Geometry: final body of the model. Coordinates: model frame, mm. A direction names the side the tool comes from. Give positions to 0.01 mm unless a question says otherwise; leave off trailing zeros. Use one line per item in the form item = value.
```python
from build123d import *

# Parameters (mm, degrees)
SKETCH_1_R      = 2.103037388
EXTRUDE_1_DEPTH = 330


with BuildPart() as part:
    # 草图1 → 凸台-拉伸1 (new body)
    with BuildSketch(Plane.XY):
        with BuildLine():
            Line((-32.248557314, -0.229845073), (-32.248557314, -1.030984477))
            Line((-32.248557314, -1.030984477), (-33.250003689, -1.030984477))
            Line((-33.250003689, -1.030984477), (-33.250003689, -6.238394755))
            ThreePointArc((-33.250003689, -6.238394755), (-32.949991565, -6.938952391), (-32.24382973, -7.225524788))
            Line((-32.24382973, -7.225524788), (-27.078556151, -7.225524788))
            Line((-27.078556151, -7.225524788), (-27.078556151, -6.224078413))
            Line((-27.078556151, -6.224078413), (-26.277399051, -6.224078413))
            Line((-26.277399051, -6.224078413), (-26.277399051, -5.212715786))
            Line((-26.277399051, -5.212715786), (-29.27300496, -5.212715786))
            Line((-29.27300496, -5.212715786), (-29.27300496, -4.211495229))
            Line((-29.27300496, -4.211495229), (-26.279632969, -1.225390538))
            Line((-26.279632969, -1.225390538), (-20.24902045, -1.225390538))
            Line((-20.24902045, -1.225390538), (-17.255648459, -4.211495229))
            Line((-17.255648459, -4.211495229), (-17.255648459, -5.212715786))
            Line((-17.255648459, -5.212715786), (-20.251254368, -5.212715786))
            Line((-20.251254368, -5.212715786), (-20.251254368, -6.224078413))
            Line((-20.251254368, -6.224078413), (-19.450097268, -6.224078413))
            Line((-19.450097268, -6.224078413), (-19.450097268, -7.225524788))
            Line((-19.450097268, -7.225524788), (-7.064233131, -7.225524788))
            Line((-7.064233131, -7.225524788), (-7.064233131, -6.224078413))
            Line((-7.064233131, -6.224078413), (-6.263076031, -6.224078413))
            Line((-6.263076031, -6.224078413), (-6.263076031, -5.212715786))
            Line((-6.263076031, -5.212715786), (-9.25868194, -5.212715786))
            Line((-9.25868194, -5.212715786), (-9.25868194, -4.211495229))
            Line((-9.25868194, -4.211495229), (-6.265309949, -1.225390538))
            Line((-6.265309949, -1.225390538), (-0.234697429, -1.225390538))
            Line((-0.234697429, -1.225390538), (2.758674561, -4.211495229))
            Line((2.758674561, -4.211495229), (2.758674561, -5.212715786))
            Line((2.758674561, -5.212715786), (-0.236931348, -5.212715786))
            Line((-0.236931348, -5.212715786), (-0.236931348, -6.224078413))
            Line((-0.236931348, -6.224078413), (0.564225752, -6.224078413))
            Line((0.564225752, -6.224078413), (0.564225752, -7.225524788))
            Line((0.564225752, -7.225524788), (12.945482254, -7.225524788))
            Line((12.945482254, -7.225524788), (12.945482254, -6.219120287))
            Line((12.945482254, -6.219120287), (13.751246989, -6.219120287))
            Line((13.751246989, -6.219120287), (13.751246989, -5.212715786))
            Line((13.751246989, -5.212715786), (10.755641081, -5.212715786))
            Line((10.755641081, -5.212715786), (10.755641081, -4.211495229))
            Line((10.755641081, -4.211495229), (13.749013071, -1.225390538))
            Line((13.749013071, -1.225390538), (19.779625591, -1.225390538))
            Line((19.779625591, -1.225390538), (22.772997581, -4.211495229))
            Line((22.772997581, -4.211495229), (22.772997581, -5.212715786))
            Line((22.772997581, -5.212715786), (19.772784037, -5.212715786))
            Line((19.772784037, -5.212715786), (19.772784037, -6.219120287))
            Line((19.772784037, -6.219120287), (20.573941137, -6.219120287))
            Line((20.573941137, -6.219120287), (20.573941137, -7.225524788))
            Line((20.573941137, -7.225524788), (25.743822351, -7.225524788))
            ThreePointArc((25.743822351, -7.225524788), (26.449984187, -6.938952391), (26.749996311, -6.238394755))
            Line((26.749996311, -6.238394755), (26.749996311, -1.030984477))
            Line((26.749996311, -1.030984477), (25.748549936, -1.030984477))
            Line((25.748549936, -1.030984477), (25.748549936, -0.229827377))
            Line((25.748549936, -0.229827377), (24.761302481, -0.229827377))
            Line((24.761302481, -0.229827377), (24.761302481, -3.234203038))
            Line((24.761302481, -3.234203038), (23.759856106, -3.234203038))
            Line((23.759856106, -3.234203038), (20.770104831, -0.237175589))
            Line((20.770104831, -0.237175589), (20.770104831, 5.786126014))
            Line((20.770104831, 5.786126014), (23.759856106, 8.783153462))
            Line((23.759856106, 8.783153462), (24.761302481, 8.783153462))
            Line((24.761302481, 8.783153462), (24.761302481, 5.778777801))
            Line((24.761302481, 5.778777801), (25.748549936, 5.778777801))
            Line((25.748549936, 5.778777801), (25.748549936, 6.579934901))
            Line((25.748549936, 6.579934901), (26.749996311, 6.579934901))
            Line((26.749996311, 6.579934901), (26.749996311, 11.768212512))
            ThreePointArc((26.749996311, 11.768212512), (26.456722319, 12.481138347), (25.743822351, 12.774475212))
            Line((25.743822351, 12.774475212), (20.573941137, 12.774475212))
            Line((20.573941137, 12.774475212), (20.573941137, 11.768070711))
            Line((20.573941137, 11.768070711), (19.772784037, 11.768070711))
            Line((19.772784037, 11.768070711), (19.772784037, 10.761666211))
            Line((19.772784037, 10.761666211), (22.772997581, 10.761666211))
            Line((22.772997581, 10.761666211), (22.772997581, 9.760445653))
            Line((22.772997581, 9.760445653), (19.779625591, 6.774340962))
            Line((19.779625591, 6.774340962), (13.749013071, 6.774340962))
            Line((13.749013071, 6.774340962), (10.755641081, 9.760445653))
            Line((10.755641081, 9.760445653), (10.755641081, 10.761666211))
            Line((10.755641081, 10.761666211), (13.746639354, 10.761666211))
            Line((13.746639354, 10.761666211), (13.746639354, 11.768070711))
            Line((13.746639354, 11.768070711), (12.945482254, 11.768070711))
            Line((12.945482254, 11.768070711), (12.945482254, 12.774475212))
            Line((12.945482254, 12.774475212), (0.564225752, 12.774475212))
            Line((0.564225752, 12.774475212), (0.564225752, 11.773028837))
            Line((0.564225752, 11.773028837), (-0.236931348, 11.773028837))
            Line((-0.236931348, 11.773028837), (-0.236931348, 10.761666211))
            Line((-0.236931348, 10.761666211), (2.758674561, 10.761666211))
            Line((2.758674561, 10.761666211), (2.758674561, 9.760445653))
            Line((2.758674561, 9.760445653), (-0.234697429, 6.774340962))
            Line((-0.234697429, 6.774340962), (-6.265309949, 6.774340962))
            Line((-6.265309949, 6.774340962), (-9.25868194, 9.760445653))
            Line((-9.25868194, 9.760445653), (-9.25868194, 10.761666211))
            Line((-9.25868194, 10.761666211), (-6.263076031, 10.761666211))
            Line((-6.263076031, 10.761666211), (-6.263076031, 11.773028837))
            Line((-6.263076031, 11.773028837), (-7.064233131, 11.773028837))
            Line((-7.064233131, 11.773028837), (-7.064233131, 12.774475212))
            Line((-7.064233131, 12.774475212), (-19.450097268, 12.774475212))
            Line((-19.450097268, 12.774475212), (-19.450097268, 11.773028837))
            Line((-19.450097268, 11.773028837), (-20.251254368, 11.773028837))
            Line((-20.251254368, 11.773028837), (-20.251254368, 10.761666211))
            Line((-20.251254368, 10.761666211), (-17.255648459, 10.761666211))
            Line((-17.255648459, 10.761666211), (-17.255648459, 9.760445653))
            Line((-17.255648459, 9.760445653), (-20.24902045, 6.774340962))
            Line((-20.24902045, 6.774340962), (-26.279632969, 6.774340962))
            Line((-26.279632969, 6.774340962), (-29.27300496, 9.760445653))
            Line((-29.27300496, 9.760445653), (-29.27300496, 10.761666211))
            Line((-29.27300496, 10.761666211), (-26.277399051, 10.761666211))
            Line((-26.277399051, 10.761666211), (-26.277399051, 11.773028837))
            Line((-26.277399051, 11.773028837), (-27.078556151, 11.773028837))
            Line((-27.078556151, 11.773028837), (-27.078556151, 12.774475212))
            Line((-27.078556151, 12.774475212), (-32.24382973, 12.774475212))
            ThreePointArc((-32.24382973, 12.774475212), (-32.956729698, 12.481138347), (-33.250003689, 11.768212512))
            Line((-33.250003689, 11.768212512), (-33.250003689, 6.560802234))
            Line((-33.250003689, 6.560802234), (-32.248557314, 6.560802234))
            Line((-32.248557314, 6.560802234), (-32.248557314, 5.759645134))
            Line((-32.248557314, 5.759645134), (-31.261309859, 5.759645134))
            Line((-31.261309859, 5.759645134), (-31.261309859, 8.764020795))
            Line((-31.261309859, 8.764020795), (-30.259863484, 8.764020795))
            Line((-30.259863484, 8.764020795), (-27.27011221, 5.766993347))
            Line((-27.27011221, 5.766993347), (-27.27011221, -0.237175589))
            Line((-27.27011221, -0.237175589), (-30.259863484, -3.234203038))
            Line((-30.259863484, -3.234203038), (-31.261309859, -3.234203038))
            Line((-31.261309859, -3.234203038), (-31.261309859, -0.229845073))
            Line((-31.261309859, -0.229845073), (-32.248557314, -0.229845073))
        make_face()
        with Locations((-3.250003689, 2.774475212)):
            Circle(SKETCH_1_R, mode=Mode.SUBTRACT)
        with Locations((-23.250003689, 2.774475212)):
            Circle(SKETCH_1_R, mode=Mode.SUBTRACT)
        with Locations((16.749996311, 2.774475212)):
            Circle(SKETCH_1_R, mode=Mode.SUBTRACT)
        Polygon((-19.258541209, 5.786126014), (-19.258541209, -0.237175589), (-15.26734356, -4.238086639), (-15.26734356, -5.22228212), (-11.246986839, -5.22228212), (-11.246986839, -4.238086639), (-7.25578919, -0.237175589), (-7.25578919, 2.774475212), (-7.25578919, 5.786126014), (-11.246986839, 9.787037063), (-11.246986839, 10.771232544), (-15.26734356, 10.771232544), (-15.26734356, 9.787037063), align=None, mode=Mode.SUBTRACT)
        Polygon((4.74697946, -5.22228212), (8.767336181, -5.22228212), (8.767336181, -4.238086639), (12.758533831, -0.237175589), (12.758533831, 2.774475212), (12.758533831, 5.786126014), (8.767336181, 9.787037063), (8.767336181, 10.771232544), (4.74697946, 10.771232544), (4.74697946, 9.787037063), (0.755781811, 5.786126014), (0.755781811, 2.774475212), (0.755781811, -0.237175589), (4.74697946, -4.238086639), align=None, mode=Mode.SUBTRACT)
    extrude(amount=EXTRUDE_1_DEPTH)


solid = part.part
```
(1) Cut plane A-A (z = 140). Give the number of separate pieces and of enclosed holes in the cut face, plus the area to 3 significant figures.
Solution:
separate_pieces = 1
enclosed_holes = 5
area = 448 mm2
(2) Pin query (flat end, axial travel): P1, Ø0.6, axis at x = -6.5, z = 119.5, coming from the +Y side; P2, Ø6, axis at y = 3, z = 238.5, coming from the +X side; P3, Ø1.5, axis at x = -26, z = 156.5, coming from the -Y side. Return the tip coordinate at first contact, or that it passes through.
Solution:
P1 = 11.77
P2 = 25.75
P3 = -6.22
(3) Pull-direction query (X, two-part tool) for faces 1 (the face through (-23, 6.774, 163)), 2 (the face through (-27.27, 3, 163)), 3 (the face through (-13, -7.226, 163)), 4 (the face through (26.75, -4, 163)); classes: released by +X, released by -X, zero draft, split by the parting line, or undercut.
Solution:
face_1 = undercut
face_2 = released by -X
face_3 = zero draft
face_4 = released by +X
(4) Material intervals for L1, parallel to X at y = 3, z = 134; L2, parallel to X at y = 5.5, z = 79; L3, parallel to Y at x = -13, z = 275, sorted ascending. Write a range as from..to.
Solution:
L1 = -27.27..-25.34, -21.16..-19.26, -7.26..-5.34, -1.16..0.76, 12.76..14.66, 18.84..20.77
L2 = -27.27..-19.26, -7.26..0.76, 12.76..20.77
L3 = -7.23..-5.22, 10.77..12.77
(5) Access query for faces 5 (the face through (-7.256, 3, 163)), 6 (the face through (-3, 6.774, 163)), 7 (the face through (-23, -1.225, 163)), 8 (the face through (20.77, 3, 163)). Directions: +Z, -Z, +X, -X, +Y, -Y. A direction counts if a zero-diameter tool reaches every point of the face in a straight line with its end or side. Return the directions, or none.
Solution:
face_5 = +Z, -Z
face_6 = +Z, -Z, +Y
face_7 = +Z, -Z, -Y
face_8 = +Z, -Z, +X
